Input: part model. Units: mm. Frame: model coordinates. Round coordinates to 2 decimals unless told otherwise and drop trailing zeros. Write each loop counter-clockwise with the first axis right and the second up, starting at its lowest first coordinate (ties: lowest second). Pieces come first, ordered by that corner, then holes. Notation, with made-up numbers: (28, 88.25) -> (49, 88.25) arc R22 cw to (49, 121.25) -> close; hole circle Ø9 at (-17, 25). An arc over 180 degrees is marked (long way). Use CSV: the item, a comma, the result in double quotes.
```python
from build123d import *

# Parameters (mm, degrees)
F0_W     = 29.9564684167
F0_H     = 43
F0_R     = 5.425
F0_R_2   = 5.95
F1_DEPTH = 10
F0_W_2   = 18.5217657917
F2_DEPTH = 10
F0_R_3   = 3.415
F3_DEPTH = 10
F4_DEPTH = 10
F6_R     = 2.5
F7_DEPTH = 5
F7_TAPER = 5
F8_R     = 5


with BuildPart() as f1:
    # F0 (on Top) → F1 (new body)
    with BuildSketch(Plane.XY):
        with Locations((0, -12)):
            Rectangle(F0_W, F0_H)
        with Locations((0, -25.365)):
            Circle(F0_R, mode=Mode.SUBTRACT)
        Circle(F0_R_2, mode=Mode.SUBTRACT)
    extrude(amount=F1_DEPTH)

    # F0 (on Top) → F2 (join)
    with BuildSketch(Plane.XY):
        with Locations((-24.2391171042, -12)):
            Rectangle(F0_W_2, F0_H)
        with Locations((-25.365, 0)):
            Circle(F0_R, mode=Mode.SUBTRACT)
        with Locations((24.2391171042, -12)):
            Rectangle(F0_W_2, F0_H)
        with Locations((25.365, 0)):
            Circle(F0_R, mode=Mode.SUBTRACT)
    extrude(amount=F2_DEPTH)

    # F0 (on Top) → F3 (join)
    with BuildSketch(Plane.XY):
        with Locations((-25.365, 0)):
            Circle(F0_R)
        with Locations((-25.365, 0)):
            Circle(F0_R_3, mode=Mode.SUBTRACT)
        with Locations((25.365, 0)):
            Circle(F0_R)
        with Locations((25.365, 0)):
            Circle(F0_R_3, mode=Mode.SUBTRACT)
        with Locations((0, -25.365)):
            Circle(F0_R)
        with Locations((0, -25.365)):
            Circle(F0_R_3, mode=Mode.SUBTRACT)
    extrude(amount=F3_DEPTH)

    # F0 (on Top) → F4 (join)
    with BuildSketch(Plane.XY):
        with Locations((24.2391171042, -12)):
            Rectangle(F0_W_2, F0_H)
        with Locations((25.365, 0)):
            Circle(F0_R, mode=Mode.SUBTRACT)
        with Locations((-24.2391171042, -12)):
            Rectangle(F0_W_2, F0_H)
        with Locations((-25.365, 0)):
            Circle(F0_R, mode=Mode.SUBTRACT)
    extrude(amount=F4_DEPTH)

    # F6 (on face) → F7 (join)
    with BuildSketch(Plane.XY.offset(10)):
        with Locations((-23.62, -23.62)):
            Circle(F6_R)
        with Locations((23.62, -23.62)):
            Circle(F6_R)
    extrude(amount=F7_DEPTH, taper=F7_TAPER)

    # F8
    f8_edges = [f1.edges().sort_by_distance(p)[0] for p in [
        (-33.5, -33.5, 5),
        (33.5, -33.5, 5),
        (33.5, 9.5, 5),
        (-33.5, 9.5, 5),
    ]]
    fillet(f8_edges, radius=F8_R)


solid = f1.part
```
Item 1: Section query D-D on z = 13.5. Return the cut outline in (x, y).
Worked answers:
outline,"circle Ø4.39 at (-23.62, -23.62); circle Ø4.39 at (23.62, -23.62)"
Item 2: First-contact query: pin 1 Ø11 at (x, y) = (25.365, 0) entering from +Z. Flat tip, straight axial feed; report the tip coordinate or a pass-through.
Worked answers:
pin 1,"stops at z = 10"
Item 3: Pull-direction query (Y, two-part tool) for faces 1 (the face through (-3, -27, 5)), 2 (the face through (-22.395, -21.699, 12.535)), 3 (the face through (0, -12, 0)), 4 (the face through (-22.1, 1, 4.9)); classes: +Y half, -Y half, draft (parallel to the pull), parting line (faces both ways), or undercut.
Worked answers:
face 1,"undercut"
face 2,"parting line"
face 3,"draft"
face 4,"undercut"
Item 4: Line query: line 1 (Y direction, x = 0, z = 5); line 2 (Y direction, x = -25.5, z = 9.75); line 3 (Z direction, x = 12.5, y = -31). Output: solid intervals per line, ascending.
Worked answers:
line 1,"y = -33.5 to -28.78, -21.95 to -5.95, 5.95 to 9.5"
line 2,"y = -33.5 to -3.41, 3.41 to 9.5"
line 3,"z = 0 to 10"
Item 5: Section query C-C on x = -23.62. Return the cut outline in (y, z), plus the area to 3 significant figures.
Worked answers:
outline,"(-33.5, 0) -> (-2.94, 0) -> (-2.94, 10) -> (-21.12, 10) -> (-21.56, 15) -> (-25.68, 15) -> (-26.12, 10) -> (-33.5, 10) -> close; (2.94, 0) -> (9.5, 0) -> (9.5, 10) -> (2.94, 10) -> close"
area,"394 mm²"
Item 6: Section query A-A on y = 0. Return the cut outline in (x, z).
Worked answers:
outline,"(-33.5, 0) -> (-28.78, 0) -> (-28.78, 10) -> (-33.5, 10) -> close; (-21.95, 0) -> (-5.95, 0) -> (-5.95, 10) -> (-21.95, 10) -> close; (5.95, 0) -> (21.95, 0) -> (21.95, 10) -> (5.95, 10) -> close; (28.78, 0) -> (33.5, 0) -> (33.5, 10) -> (28.78, 10) -> close"
Item 7: Section query B-B on y = -23.62. Return the cut outline in (x, z).
Worked answers:
outline,"(-33.5, 0) -> (-2.94, 0) -> (-2.94, 10) -> (-21.12, 10) -> (-21.56, 15) -> (-25.68, 15) -> (-26.12, 10) -> (-33.5, 10) -> close; (2.94, 0) -> (33.5, 0) -> (33.5, 10) -> (26.12, 10) -> (25.68, 15) -> (21.56, 15) -> (21.12, 10) -> (2.94, 10) -> close"
